Read the model definition and answer for the solid it produces. Units are mm, in the model's axes. Round coordinates to 2 decimals unless told otherwise and drop trailing zeros. Order: outer loops, then holes, each group sorted by start corner. A loop starts at its lowest first (then second) coordinate and runs counter-clockwise, first axis right, second up. Notation, with made-up numbers: M 80.5,-13 L 106.5,-13 A26 ccw 106.5,17 Z; hole C 12.5,76 d10. An arc over 180 degrees is marked long. Answer as CSV lines item,"result".
```python
from build123d import *

# Parameters (mm, degrees)
BODYSKE_R  = 0.6
BODY_DEPTH = 1.3


with BuildPart() as part:
    # BodySke → Body (new body)
    with BuildSketch(Plane.XY):
        with BuildLine():
            Line((0.223172324, -6.571211389), (0.325, -9.569482745))
            ThreePointArc((0.325, -9.569482745), (2.067179303, -9.349192197), (3.739828154, -8.81443761))
            ThreePointArc((3.739828154, -8.81443761), (4.145198739, -8.499227928), (4.340690441, -8.024395905))
            Line((4.340690441, -8.024395905), (4.445467219, -7.228537259))
            ThreePointArc((4.445467219, -7.228537259), (4.649323286, -6.632069256), (5.06788143, -6.160751471))
            ThreePointArc((5.06788143, -6.160751471), (0, 8.975), (-5.06788143, -6.160751471))
            ThreePointArc((-5.06788143, -6.160751471), (-4.649323286, -6.632069256), (-4.445467219, -7.228537259))
            Line((-4.445467219, -7.228537259), (-4.340690441, -8.024395905))
            ThreePointArc((-4.340690441, -8.024395905), (-4.145198739, -8.499227928), (-3.739828154, -8.81443761))
            ThreePointArc((-3.739828154, -8.81443761), (-2.067179303, -9.349192197), (-0.325, -9.569482745))
            Line((-0.325, -9.569482745), (-0.223172324, -6.571211389))
            ThreePointArc((-0.223172324, -6.571211389), (0, 6.575), (0.223172324, -6.571211389))
        make_face()
        with Locations((1.25, -8.192689195)):
            Circle(BODYSKE_R, mode=Mode.SUBTRACT)
        with Locations((-1.25, -8.192689195)):
            Circle(BODYSKE_R, mode=Mode.SUBTRACT)
    extrude(amount=-BODY_DEPTH)


solid = part.part
```
Item 1: A cutting plane is placed at D-D, the plane x = 0. Determine the outline of the cut face in (y, z) (3 decimals), and give its area (3 significant figures).
Ans:
outline,"M 6.575,-1.3 L 8.975,-1.3 L 8.975,0 L 6.575,0 Z"
area,"3.12 mm2"
Item 2: A flat-ended cylindrical pin translates along its axis: pin 1 (1.4 mm diameter, centred on x = -1.25, y = -8.19, fed in from -Z). Find the tip coordinate at first contact, or state that the pin passes through.
Ans:
pin 1,"z = -1.3"
Item 3: A cutting plane is placed at B-B, the plane x = -2.75. Determine the outline of the cut face in (y, z).
Ans:
outline,"M -9.17,-1.3 L -5.97,-1.3 L -5.97,0 L -9.17,0 Z; M 5.97,-1.3 L 8.51,-1.3 L 8.51,0 L 5.97,0 Z"
Item 4: A cutting plane is placed at A-A, the plane y = -3.25. Determine the outline of the cut face in (x, z).
Ans:
outline,"M -7.51,-1.3 L -5.72,-1.3 L -5.72,0 L -7.51,0 Z; M 5.72,-1.3 L 7.51,-1.3 L 7.51,0 L 5.72,0 Z"
Item 5: Find the intervals of material crossed by probe 1 along Y at (x, z) = (-1.25, -0.95); probe 2 along Y at (x, z) = (-1, -0.2); probe 3 along X at (y, z) = (4.75, -0.85), in increasing order. Write a range as [from, to].
Ans:
probe 1,"[-9.49, -8.79], [-7.59, -6.46], [6.46, 8.88]"
probe 2,"[-9.52, -8.74], [-7.65, -6.5], [6.5, 8.92]"
probe 3,"[-7.3, -4.55], [4.55, 7.3]"
Item 6: Determine the mould class of faces 1 (the face through (0, 7, -1.3)), 2 (the face through (-1.33, -7.6, -0.64)), 3 (the face through (-4.654, -6.624, -0.641)) for opening direction X: +X half, -X half, draft (parallel to the pull), parting line (faces both ways), or undercut.
Ans:
face 1,"draft"
face 2,"undercut"
face 3,"-X half"
Item 7: A cutting plane is placed at C-C, the plane z = -0.45. Determine the outline of the cut face in (x, y) (3 decimals), and give its area (3 significant figures).
Ans:
outline,"M -5.068,-6.161 A1.599 cw -4.445,-7.229 L -4.341,-8.024 A1 ccw -3.74,-8.814 A9.575 ccw -0.325,-9.569 L -0.223,-6.571 A6.575 cw long 0.223,-6.571 L 0.325,-9.569 A9.575 ccw 3.74,-8.814 A1 ccw 4.341,-8.024 L 4.445,-7.229 A1.599 cw 5.068,-6.161 A8.416 ccw long Z; hole C -1.25,-8.193 d1.2; hole C 1.25,-8.193 d1.2"
area,"98.4 mm2"
